```python
from build123d import *

# Parameters (mm, degrees)
BOSS_EXTRUDE1_DEPTH = 1.8
SKETCH2_R           = 1
BOSS_EXTRUDE2_DEPTH = 3
BOSS_EXTRUDE2_DRAFT = -18.434


with BuildPart() as part:
    # Sketch1 → Boss-Extrude1 (new body)
    with BuildSketch(Plane.XY):
        with BuildLine():
            Line((-33.5, -21.5), (33.5, -21.5))
            ThreePointArc((33.5, -21.5), (34.207106781, -21.207106781), (34.5, -20.5))
            Line((34.5, -20.5), (34.5, 20.5))
            ThreePointArc((34.5, 20.5), (34.207106781, 21.207106781), (33.5, 21.5))
            Line((33.5, 21.5), (-33.5, 21.5))
            ThreePointArc((-33.5, 21.5), (-34.207106781, 21.207106781), (-34.5, 20.5))
            Line((-34.5, 20.5), (-34.5, -20.5))
            ThreePointArc((-34.5, -20.5), (-34.207106781, -21.207106781), (-33.5, -21.5))
        make_face()
    extrude(amount=BOSS_EXTRUDE1_DEPTH)


with BuildPart() as boss_extrude2_tool:
    # Sketch2 → Boss-Extrude2 (with draft: the straight prism first)
    with BuildSketch(Plane.XY.offset(1.8)):
        with Locations((32.5, 0)):
            Circle(SKETCH2_R)
    extrude(amount=BOSS_EXTRUDE2_DEPTH)
    # Boss-Extrude2: the draft: its side faces are tilted about the plane it starts from
    boss_extrude2_sides = [boss_extrude2_tool.faces().sort_by_distance(p)[0] for p in [
        (31.5, 0, 3.3),
    ]]
    draft(boss_extrude2_sides, Plane.XY.offset(1.8), BOSS_EXTRUDE2_DRAFT)


with BuildPart() as part_1:
    add(part.part)

    # Boss-Extrude2: add boss_extrude2_tool
    add(boss_extrude2_tool.part)


solid = part_1.part
```
Verification items for the finished model (mm, model axes). Coordinates: 2 decimals unless noted, no trailing zeros. Write each loop counter-clockwise with the first axis right and the second up, starting at its lowest first coordinate (ties: lowest second). Pieces come first, ordered by that corner, then holes. Notation, with made-up numbers: M 74,14.5 L 99,14.5 A19 ccw 99,40.5 Z; hole C -16.5,78 d11. An arc over 180 degrees is marked long. One line per item, written item: value.
Item 1: Section check D-D, the plane y = -6. Record the boundary of the cut face in (x, z), plus the area to 3 significant figures.
Check sheet entries:
outline: M -34.5,0 L 34.5,0 L 34.5,1.8 L -34.5,1.8 Z
area: 124 mm^2
Item 2: Mould release check, pull along Z, two halves, no side actions. Record for faces 1 (the flat face through (0, 0, 0)), 2 (the conical face through (31.4, -0.84, 2.95)), 3 (the flat face through (32, 0, 4.8)), 4 (the flat face through (-34.5, 0, 1)): pulls with the +Z half, pulls with the -Z half, needs draft (parallel to the pull), parting line crosses it, or undercut.
Check sheet entries:
face 1: pulls with the -Z half
face 2: undercut
face 3: pulls with the +Z half
face 4: needs draft
Item 3: Section check B-B, the plane y = 0. Record the boundary of the cut face in (x, z).
Check sheet entries:
outline: M -34.5,0 L 34.5,0 L 34.5,1.8 L 33.5,1.8 L 34.5,4.8 L 30.5,4.8 L 31.5,1.8 L -34.5,1.8 Z
Item 4: Section check A-A, the plane x = 32.5. Record the boundary of the cut face in (y, z), plus the area to 3 significant figures.
Check sheet entries:
outline: M -21.5,0 L 21.5,0 L 21.5,1.8 L 1,1.8 L 2,4.8 L -2,4.8 L -1,1.8 L -21.5,1.8 Z
area: 86.4 mm^2
Item 5: Gauge pin test, flat end, axial feed: pin 1 Ø5 at (x, y) = (-18, -1.5) entering from +Z. Record the tip position at first contact, or that the pin passes through.
Check sheet entries:
pin 1: stops at z = 1.8
Item 6: Scan lines: line 1 along Z through (x, y) = (11, 12.5); line 2 along X through (y, z) = (1, 2.35); line 3 along X through (y, z) = (0.5, 4.5). Record each from-to range of solid material in increasing order.
Check sheet entries:
line 1: z = 0 to 1.8
line 2: x = 31.87 to 33.13
line 3: x = 30.67 to 34.33
Item 7: Section check C-C, the plane z = 3.65. Record the boundary of the cut face in (x, y), plus the area to 3 significant figures.
Check sheet entries:
outline: C 32.5,0 d3.23
area: 8.21 mm^2
